```python
from build123d import *

# Parameters (mm, degrees)
F0_R      = 15.875
F1_DEPTH  = 25.4
F2_W      = 49.386511
F2_H      = 19.034712
F3_DEPTH  = 19.05
F4_R      = 1.8288
F5_DEPTH  = 6.351
F6_R      = 4.7625
F7_DEPTH  = 12.7
F8_R      = 3.175
F9_DEPTH  = 23.0124
F10_R     = 1.35255
F11_DEPTH = 14.2885


with BuildPart() as f1:
    # F0 (on Right) → F1 (new body)
    with BuildSketch(Plane.YZ):
        Circle(F0_R)
    extrude(amount=F1_DEPTH)

    # F2 (on face) → F3 (cut)
    with BuildSketch(Plane.YZ.offset(25.4)):
        with Locations((-1.538695, -7.929856)):
            Rectangle(F2_W, F2_H)
    extrude(amount=-F3_DEPTH, mode=Mode.SUBTRACT)

    # F4 (on face) → F5 (cut, through all)
    with BuildSketch(Plane.YZ.offset(6.35)):
        Circle(F4_R)
    extrude(amount=-F5_DEPTH, mode=Mode.SUBTRACT)

    # F6 (on face) → F7 (cut)
    with BuildSketch(Plane.YZ.offset(25.4)):
        Circle(F6_R)
    extrude(amount=-F7_DEPTH, mode=Mode.SUBTRACT)

    # F8 (on face) → F9 (cut)
    with BuildSketch(Plane.YZ.offset(25.4)):
        Circle(F8_R)
    extrude(amount=-F9_DEPTH, mode=Mode.SUBTRACT)

    # F10 (on face) → F11 (cut, through all)
    with BuildSketch(Plane(origin=(0, 0, 1.5875), x_dir=(1, 0, 0), z_dir=(0, 0, -1))):
        with Locations((19.05, 10.142777)):
            Circle(F10_R)
        with Locations((19.05, -10.142777)):
            Circle(F10_R)
    extrude(amount=-F11_DEPTH, mode=Mode.SUBTRACT)


solid = f1.part
```
Can you work these out from the model? Positions are in its coordinate system, mm. A direction names the side the tool comes from. Give positions to 0.01 mm unless a question says otherwise; leave off trailing zeros. Loops run counter-clockwise (first coordinate to the right, second up) from the corner with the lowest first, then second, coordinate; pieces in that order, holes last. Notation, with made-up numbers: M 42.25,-6 L 56.25,-6 A5 cw 56.25,-1 Z; hole C -27.75,-27 d1. An arc over 180 degrees is marked long. Answer in a Markdown table with one row per item.
1. If I drill on line 1 along Y through (x, z) = (19.05, 10.5); line 2 along Z through (x, y) = (1.75, 0) (3 decimals); line 3 along Z through (x, y) = (5.25, 0) (3 decimals), over which ranges is the centre line in solid material (lowest first)?
Taken from the geometry:
| item | result |
|---|---|
| line 1 | y = -11.91 to -11.5, -8.79 to 8.79, 11.5 to 11.91 |
| line 2 | z = -15.875 to -1.829, 1.829 to 15.875 |
| line 3 | z = -15.875 to -3.175, 3.175 to 15.875 |
2. Which directions (+Z, -Z, +X, -X, +Y, -Y) give clear straight access to the entire face, cutting with the end or side of a thin tool? Please do faces 5 (the flat face through (2.388, 1.4, -1.4)), 6 (the flat face through (16, 9, 1.587)), 7 (the flat face through (12.7, 0, 4)).
Taken from the geometry:
| item | result |
|---|---|
| face 5 | +X |
| face 6 | -Z, +X, +Y, -Y |
| face 7 | -Z, +X |
3. Suppose I cut it at D-D on z = 8. Write out the boundary of the cut face in (x, y), plus the area to 3 significant figures.
Taken from the geometry:
| item | result |
|---|---|
| outline | M 0,-13.71 L 25.4,-13.71 L 25.4,13.71 L 0,13.71 Z; hole C 19.05,-10.14 d2.71; hole C 19.05,10.14 d2.71 |
| area | 685 mm² |
4. Thinking about a two-plate mould opening in Y: for faces 1 (the cylindrical face through (9.7, -2.07, 15.74)), 2 (the cylindrical face through (1.211, -1.451, -1.113)), 3 (the flat face through (6.35, 0, -5)), 4 (the cylindrical face through (6.47, -0.41, 3.15)), which applies, released by +Y, released by -Y, zero draft, split by the parting line, or undercut?
Taken from the geometry:
| item | result |
|---|---|
| face 1 | split by the parting line |
| face 2 | undercut |
| face 3 | zero draft |
| face 4 | undercut |
5. Suppose I cut it at B-B on z = 0. Write out the boundary of the cut face in (x, y) (3 decimals).
Taken from the geometry:
| item | result |
|---|---|
| outline | M 0,-15.875 L 6.35,-15.875 L 6.35,-3.175 L 2.388,-3.175 L 2.388,-1.829 L 0,-1.829 Z; M 0,1.829 L 2.388,1.829 L 2.388,3.175 L 6.35,3.175 L 6.35,15.875 L 0,15.875 Z |
6. For pin 1 Ø6.5 at (x, y) = (15.5, -12) entering from -Z; pin 2 Ø1 at (y, z) = (9, 11.5) entering from -X; pin 3 Ø2 at (x, y) = (11.5, 4.5) entering from +Z; pin 4 Ø2 at (x, z) = (13, 5) entering from -Y, each with a flat end and sliding along its axis, tell me the tip position at first contact or that it passes through.
Taken from the geometry:
| item | result |
|---|---|
| pin 1 | stops at z = 1.59 |
| pin 2 | stops at x = 0 |
| pin 3 | stops at z = 15.48 |
| pin 4 | stops at y = -15.36 |
7. Suppose I cut it at C-C on x = 19.05. Count the separate pieces of the cut face and the enclosed holes in it, plus the area to 3 significant figures.
Taken from the geometry:
| item | result |
|---|---|
| separate pieces | 3 |
| enclosed holes | 0 |
| area | 268 mm² |
